Design review of the part built by this model. Coordinates are the model's own, in mm. A direction names the side the tool comes from. Give positions to 0.01 mm unless a question says otherwise; leave off trailing zeros. Order: outer loops, then holes, each group sorted by start corner. A loop starts at its lowest first (then second) coordinate and runs counter-clockwise, first axis right, second up. Notation, with made-up numbers: (83, 71) -> (130, 71) arc R10 cw to (130, 75) -> close; hole circle Ø7 at (1, 87). An arc over 180 degrees is marked (long way). One line per item, written item: value. Start each with the question number.
1) Consider section A-A (x = 30). State the section outline as (y, z) points.
2) Tool access review of faces 1 (the face through (33.02, -16, 17)), 2 (the face through (17, -3.81, 16)): name each direction out of +Z, -Z, +X, -X, +Y, -Y from which nothing blocks a thin tool from reaching the whole face with its end or side.
3) For pin 1 (8 mm diameter, centred on x = 19, y = -14, fed in from +Z); pin 2 (5 mm diameter, centred on x = 20, y = -30, fed in from +Z); pin 3 (7.5 mm diameter, centred on x = 17, z = 21.5, fed in from -Y), all flat-tipped, find the tip position at first contact; note any pin that passes through.
4) Wall thickness on line 1 along Z through (x, y) = (20.5, -12); line 2 along Z through (x, y) = (28.5, -23.5); line 3 along Y through (x, z) = (16, 22.5): over which ranges is each line inside the solid? List them lowest first. Write a range as from..to.
5) The part is to be moulded in two halves that separate along Z. For faces 3 (the face through (23.6, -18.8, 19.3)), 4 (the face through (16, 0, 16)), 5 (the face through (17, -17, 3.81)), say which applies: released by +Z, released by -Z, zero draft, split by the parting line, or undercut.
6) Consider section B-B (y = -26). State how many separate pieces and enclosed holes the cut face has, plus the area to 3 significant figures.
from build123d import *

# Parameters (mm, degrees)
F1_DEPTH = 33.02
F2_R     = 2.54
F4_DEPTH = 33.021
F7_DEPTH = 45.72


with BuildPart() as f1:
    # F0 (on Right) → F1 (new body)
    with BuildSketch(Plane.YZ):
        Polygon((-38.1, 0), (0, 0), (0, 38.1), align=None)
    extrude(amount=F1_DEPTH)

    # F2
    f2_edges = [f1.edges().sort_by_distance(p)[0] for p in [
        (16.51, 0, 38.1),
        (16.51, -38.1, 0),
    ]]
    fillet(f2_edges, radius=F2_R)

    # F3 (on face) → F4 (cut, through all)
    with BuildSketch(Plane.YZ.offset(33.02)):
        Polygon((-28.9018463274, 3.81), (-3.81, 3.81), (-3.81, 28.9018463274), align=None)
    extrude(amount=-F4_DEPTH, mode=Mode.SUBTRACT)

    # F6 (on offset) → F7 (cut)
    with BuildSketch(Plane.XY.offset(50.8)):
        with BuildLine():
            add(Edge.make_bspline(
                [(16.1240324378, -27.884254232), (28.7915867598, -27.884254232), (22.4578095988, -13.4440287948), (16.1240324378, 0.9961966425), (9.7902552768, -13.4440287948), (3.4564781158, -27.884254232), (16.1240324378, -27.884254232)],
                knots=[0, 0, 0, 2.0943951024, 2.0943951024, 4.1887902048, 4.1887902048, 6.2831853072, 6.2831853072, 6.2831853072], degree=2, weights=[1, 0.5, 1, 0.5, 1, 0.5, 1]))
        make_face()
    extrude(amount=-F7_DEPTH, mode=Mode.SUBTRACT)


solid = f1.part
Checked values:
1. outline: (-33.76, 4.34) arc R2.54 ccw to (-31.97, 0) -> (0, 0) -> (0, 31.97) arc R2.54 ccw to (-4.34, 33.76) -> close; hole (-28.9, 3.81) -> (-3.81, 3.81) -> (-3.81, 28.9) -> close
2. face 1: +Z, -Z, +X, +Y, -Y
2. face 2: +X, -X
3. pin 1: stops at z = 27.96
3. pin 2: stops at z = 10.6
3. pin 3: stops at y = -10.77
4. line 1: z = 0..3.81
4. line 2: z = 0..3.81, 9.21..14.6
4. line 3: y = -3.81..0
5. face 3: released by +Z
5. face 4: zero draft
5. face 5: undercut
6. separate pieces: 3
6. enclosed holes: 0
6. area: 257 mm^2
